```python
from build123d import *

# Parameters (mm, degrees)
SKETCH2_W                    = 3.175
SKETCH2_H                    = 19.05
F_1_8_0_125_DIAMETER_HOLE1_D = 3.175
F_1_8_0_125_DIAMETER_HOLE2_D = 3.175
FILLET1_R                    = 12.7
FILLET2_R                    = 6.35
CHAMFER3_SIZE                = 0.762
CHAMFER2_SIZE                = 0.254


with BuildPart() as part:
    # Sweep1: sweep along a path in Sketch1
    with BuildLine(Plane.XY) as sweep1_path:
        Line((0, 0), (0, -47.5145354))
        Line((0, -47.5145354), (33.61082832, -105.730197734))
        Line((33.61082832, -105.730197734), (68.53582832, -105.730197734))
    # Sketch2 → Sweep1 (sweep)
    with BuildSketch(Plane(origin=(0, 0, 0), x_dir=(1, 0, 0), z_dir=(0, 1, 0))):
        Rectangle(SKETCH2_W, SKETCH2_H)
    sweep(path=sweep1_path.line, transition=Transition.RIGHT)

    # 1/8 (0.125) Diameter Hole1 (through all)
    with Locations(Plane(origin=(1.5875, 0, 0), x_dir=(0, 0, -1), z_dir=(1, 0, 0))):
        with Locations((0, -11.693565329), (0, -24.393565329)):
            Hole(F_1_8_0_125_DIAMETER_HOLE1_D / 2)

    # 1/8 (0.125) Diameter Hole2 (through all)
    with Locations(Plane(origin=(0, -104.142697734, 0), x_dir=(1, 0, 0), z_dir=(0, 1, 0))):
        with Locations((59.01082832, 0)):
            Hole(F_1_8_0_125_DIAMETER_HOLE2_D / 2)

    # Fillet1
    fillet1_edges = [part.edges().sort_by_distance(p)[0] for p in [
        (1.5875, -47.089166057, 0),
        (-1.5875, -47.939904743, 0),
        (32.694284767, -107.317697734, 0),
        (34.527371872, -104.142697734, 0),
    ]]
    fillet(fillet1_edges, radius=FILLET1_R)

    # Fillet2
    fillet2_edges = [part.edges().sort_by_distance(p)[0] for p in [
        (0, 0, -9.525),
        (0, 0, 9.525),
        (68.53582832, -105.730197734, -9.525),
        (68.53582832, -105.730197734, 9.525),
    ]]
    fillet(fillet2_edges, radius=FILLET2_R)

    # Chamfer3
    chamfer3_edges = [part.edges().sort_by_distance(p)[0] for p in [
        (68.53582832, -107.317697734, 0),
        (66.67595638, -107.317697734, 7.665128061),
        (66.67595638, -107.317697734, -7.665128061),
        (68.53582832, -104.142697734, 0),
        (66.67595638, -104.142697734, 7.665128061),
        (66.67595638, -104.142697734, -7.665128061),
        (1.5875, 0, 0),
        (-1.5875, 0, 0),
        (-1.5875, -25.443475, -9.525),
        (-1.5875, -25.443475, 9.525),
        (-1.5875, -1.859871939, 7.665128061),
        (-1.5875, -1.859871939, -7.665128061),
        (1.5875, -25.018105657, -9.525),
        (1.5875, -25.018105657, 9.525),
        (1.5875, -1.859871939, 7.665128061),
        (1.5875, -1.859871939, -7.665128061),
        (51.106230753, -107.317697734, -9.525),
        (51.106230753, -107.317697734, 9.525),
        (52.022774305, -104.142697734, -9.525),
        (33.676633186, -105.616220362, -9.525),
        (14.571043965, -75.927323867, -9.525),
        (17.075087517, -73.914454524, -9.525),
        (-1.154757994, -47.823951872, -9.525),
        (33.676633186, -105.616220362, -9.525),
        (14.571043965, -75.927323867, 9.525),
        (17.075087517, -73.914454524, 9.525),
        (-1.154757994, -47.823951872, 9.525),
        (33.676633186, -105.616220362, 9.525),
        (52.022774305, -104.142697734, 9.525),
        (33.676633186, -105.616220362, 9.525),
        (-1.154757994, -47.823951872, -9.525),
        (-1.154757994, -47.823951872, 9.525),
        (35.509720291, -102.441220362, 9.525),
        (35.509720291, -102.441220362, 9.525),
        (35.509720291, -102.441220362, -9.525),
        (35.509720291, -102.441220362, -9.525),
        (2.020242006, -46.973213186, 9.525),
        (2.020242006, -46.973213186, 9.525),
        (2.020242006, -46.973213186, -9.525),
        (2.020242006, -46.973213186, -9.525),
    ]]
    chamfer(chamfer3_edges, length=CHAMFER3_SIZE)

    # Chamfer2
    chamfer2_edges = [part.edges().sort_by_distance(p)[0] for p in [
        (1.5875, -24.393565329, -1.5875),
        (-1.5875, -24.393565329, -1.5875),
        (1.5875, -11.693565329, -1.5875),
        (-1.5875, -11.693565329, -1.5875),
        (60.59832832, -104.142697734, 0),
        (60.59832832, -107.317697734, 0),
    ]]
    chamfer(chamfer2_edges, length=CHAMFER2_SIZE)


solid = part.part
```
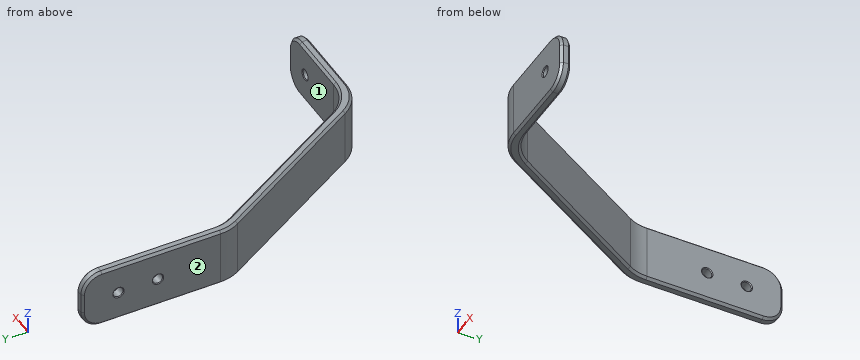
Input: part model. Units: mm. Frame: model coordinates. Face numbers are marked on the shaded views. A direction names the side the tool comes from. Coordinates: 2 decimals unless noted, no trailing zeros. Write each loop counter-clockwise with the first axis right and the second up, starting at its lowest first coordinate (ties: lowest second). Pieces come first, ordered by that corner, then holes. Notation, with made-up numbers: (-1.75, 83) - (51.25, 83) arc R26 ccw to (51.25, 122) - close; hole circle Ø3 at (-11, 2). An arc over 180 degrees is marked (long way). Put each result on its own line as item: value. Start each with the question number.
1) Cut plane C-C (z = 0). State how many separate pieces and enclosed holes the cut face has, plus the area to 3 significant figures.
2) Contact query for flat-ended pins moving along their axis: pin 1 (6 mm diameter, centred on y = -87.5, z = 3, fed in from +X); pin 2 (2 mm diameter, centred on x = 35.5, z = 4, fed in from -Y); pin 3 (10 mm diameter, centred on x = 57.5, z = 3, fed in from +Y); pin 4 (2.5 mm diameter, centred on y = -24.39, z = 0, fed in from +X). Output: stop coordinate, or through.
3) Reachability of the marked faces 1 and 2 from +Z, -Z, +X, -X, +Y, -Y: full face, straight path, thin tool, end or side. Return the list, or none.
4) Ray query, L1, parallel to Y at x = 0.65, z = 0; L2, parallel to Y at x = 0.15, z = 0; L3, parallel to Y at x = 63.5, z = -5.5. Return the intervals inside material, ascending.
5) Cut plane A-A (y = -39.5). Return the cut outline in (x, z) (1 decimal).
6) Cut plane B-B (x = 50). Return the cut outline in (y, z) (3 decimals).
Resolved:
1. separate pieces: 4
1. enclosed holes: 0
1. area: 443 mm2
2. pin 1: stops at x = 26.65
2. pin 2: stops at y = -106.82
2. pin 3: stops at y = -104.14
2. pin 4: passes through
3. face 1: +Z, -Z, +X, +Y
3. face 2: +Z, -Z, -X, +Y, -Y
4. L1: y = -51.82 to -25.98, -22.81 to -13.28, -10.11 to 0
4. L2: y = -50.95 to -25.98, -22.81 to -13.28, -10.11 to 0
4. L3: y = -107.32 to -104.14
5. outline: (-1.6, -8.8) - (-0.8, -9.5) - (0.8, -9.5) - (1.6, -8.8) - (1.6, 8.8) - (0.8, 9.5) - (-0.8, 9.5) - (-1.6, 8.8) - close
6. outline: (-107.318, -8.763) - (-106.556, -9.525) - (-104.905, -9.525) - (-104.143, -8.763) - (-104.143, 8.763) - (-104.905, 9.525) - (-106.556, 9.525) - (-107.318, 8.763) - close
